Read the model definition and answer for the solid it produces. Units are mm, in the model's axes. A direction names the side the tool comes from. Give positions to 0.01 mm unless a question says otherwise; leave off trailing zeros. Write each loop counter-clockwise with the first axis right and the second up, starting at its lowest first coordinate (ties: lowest second). Pieces come first, ordered by that corner, then holes. Notation, with made-up numbers: M 61.5,5 L 91.5,5 A14 ccw 91.5,31 Z; hole C 89.5,85 d3. An arc over 180 degrees is marked long. Use a Markdown table: item, result. Add a question column.
Item 1: Consider probe 1 along Y at (x, z) = (-8, -0.8); probe 2 along X at (y, z) = (15.75, -0.5); probe 3 along Y at (x, z) = (-11.25, -0.5). Determine where each line is inside the solid, lowest interval first. Write a range as [from, to].
Item 2: A cutting plane is placed at B-B on y = 12. Determine the outline of the cut face in (x, z).
Item 3: Given P1, Ø1.5, axis at y = 13.5, z = 2, coming from the -X side; P2, Ø3, axis at y = 8, z = 4, coming from the +X side; P3, Ø3, axis at x = -5, z = 3.5, coming from the -Y side, each flat-ended and moving along its own axis, determine where each tip first touches the part or whether it passes through.
Item 4: A cutting plane is placed at C-C on z = 4. Determine the outline of the cut face in (x, y), then the cut area to 3 significant figures.
Item 5: A cutting plane is placed at A-A on x = -8. Determine the outline of the cut face in (y, z), then the cut area to 3 significant figures.
Item 6: A cutting plane is placed at D-D on y = 15. Determine the outline of the cut face in (x, z).
Item 7: For faces 4 (the flat face through (-2.8, 12.1, -2)), 5 (the cylindrical face through (-6.44, 11.93, 4.35)), determine the directions among +Z, -Z, +X, -X, +Y, -Y from which every point of the face is accessible in a straight line to the end or side of a thin tool.
Item 8: The mould has two halves that part along X. Classify faces 1 (the cylindrical face through (-5.693, 7.564, 2.437)), 2 (the flat face through (-16.291, 10.846, -2.465)), 3 (the flat face through (-8, 12, 7)): pulls with the +X half, pulls with the -X half, needs draft (parallel to the pull), parting line crosses it, or undercut.
from build123d import *

# Parameters (mm, degrees)
EXTRUDE_1_DEPTH     = 22
SKETCH_2_R          = 5
EXTRUDE_2_DEPTH     = 7
CUT_EXTRUDE_START   = -2
SKETCH_3_R          = 8.1
SKETCH_3_R_2        = 5
CUT_EXTRUDE_1_DEPTH = 2
SKETCH_4_R          = 1.6
CUT_EXTRUDE_2_DEPTH = 31.545048699


with BuildPart() as part:
    # 草图1 → 凸台-拉伸1 (new body)
    with BuildSketch(Plane(origin=(0, 0, 0), x_dir=(1, 0, 0), z_dir=(0, 1, 0))):
        Polygon((0, 0), (-20, 0), (-12.477453102, 5), (0, 5), align=None)
    extrude(amount=EXTRUDE_1_DEPTH)

    # 草图2 → 凸台-拉伸2 (add)
    with BuildSketch(Plane.XY):
        with Locations((-8, 12)):
            Circle(SKETCH_2_R)
    extrude(amount=EXTRUDE_2_DEPTH)

    # 草图3 → 切除-拉伸1 (cut)
    with BuildSketch(Plane.XY.offset(CUT_EXTRUDE_START)):
        with Locations((-8, 12)):
            Circle(SKETCH_3_R)
        with Locations((-8, 12)):
            Circle(SKETCH_3_R_2, mode=Mode.SUBTRACT)
    extrude(amount=CUT_EXTRUDE_1_DEPTH, mode=Mode.SUBTRACT)

    # 草图4 → 切除-拉伸2 (cut, through all)
    with BuildSketch(Plane(origin=(0, 0, 0), x_dir=(1, 0, 0), z_dir=(0, 1, 0))):
        with Locations(Location((-8, -4, 0), (0, 0, 90))):
            Circle(SKETCH_4_R)
    extrude(amount=CUT_EXTRUDE_2_DEPTH, mode=Mode.SUBTRACT)


solid = part.part
Filled in:
| question | item | result |
|---|---|---|
| 1 | probe 1 | [0, 3.9], [7, 17], [20.1, 22] |
| 1 | probe 2 | [-19.25, -15.18], [-11.31, -4.69], [-0.82, 0] |
| 1 | probe 3 | [0, 4.58], [8.2, 15.8], [19.42, 22] |
| 2 | outline | M -20,0 L -12.48,-5 L 0,-5 L 0,-2 L -3,-2 L -3,7 L -13,7 L -13,-2 L -16.1,-2 L -16.1,0 Z; hole C -8,4 d3.2 |
| 3 | P1 | x = -12.94 |
| 3 | P2 | x = -3.67 |
| 3 | P3 | y = 7.23 |
| 4 | outline | M -9.6,7.26 L -9.6,16.74 A5 ccw Z; M -6.4,7.26 A5 ccw -6.4,16.74 Z |
| 4 | area | 47.1 mm² |
| 5 | outline | M 0,-5 L 22,-5 L 22,0 L 20.1,0 L 20.1,-2 L 17,-2 L 17,2.4 L 7,2.4 L 7,-2 L 3.9,-2 L 3.9,0 L 0,0 Z; M 7,5.6 L 17,5.6 L 17,7 L 7,7 Z |
| 5 | area | 136 mm² |
| 6 | outline | M -20,0 L -12.48,-5 L 0,-5 L 0,0 L -0.48,0 L -0.48,-2 L -4,-2 L -4,7 L -12,7 L -12,-2 L -15.52,-2 L -15.52,0 Z; hole C -8,4 d3.2 |
| 7 | face 4 | +Z |
| 7 | face 5 | +Y, -Y |
| 8 | face 1 | undercut |
| 8 | face 2 | pulls with the -X half |
| 8 | face 3 | needs draft |
